```python
from build123d import *

# Parameters (mm, degrees)
SKETCH1_W           = 95.25
SKETCH1_H           = 101.6
BOSS_EXTRUDE1_DEPTH = 3.175
SKETCH5_R           = 0.99949
CUT_EXTRUDE3_DEPTH  = 3.175
CIRPATTERN3_COUNT   = 2
FILLET1_R           = 2.54
CHAMFER1_SIZE       = 1.27


with BuildPart() as part:
    # Sketch1 → Boss-Extrude1 (new body)
    with BuildSketch(Plane(origin=(0, 0, 0), x_dir=(1, 0, 0), z_dir=(0, 1, 0))):
        Rectangle(SKETCH1_W, SKETCH1_H)
    extrude(amount=BOSS_EXTRUDE1_DEPTH)

    # Sketch5 → Cut-Extrude3 (cut)
    with BuildSketch(Plane(origin=(0, 3.175, 0), x_dir=(1, 0, 0), z_dir=(0, 1, 0))):
        with Locations((-38.1, -44.45)):
            Circle(SKETCH5_R)
        with Locations((38.1, -44.45)):
            Circle(SKETCH5_R)
    cut_extrude3 = extrude(amount=-CUT_EXTRUDE3_DEPTH, mode=Mode.SUBTRACT)

    # CirPattern3: Cut-Extrude3 ×2 about axis
    cirpattern3_axis = Axis((0, 0, 0), (0, 1, 0))
    for i in range(1, CIRPATTERN3_COUNT):
        add(cut_extrude3.rotate(cirpattern3_axis, i * 360 / CIRPATTERN3_COUNT), mode=Mode.SUBTRACT)

    # Fillet1
    fillet1_edges = [part.edges().sort_by_distance(p)[0] for p in [
        (47.625, 3.175, 0),
        (0, 3.175, -50.8),
        (-47.625, 3.175, 0),
        (-47.625, 1.5875, -50.8),
        (47.625, 1.5875, -50.8),
        (47.625, 1.5875, 50.8),
        (-47.625, 1.5875, 50.8),
        (0, 3.175, 50.8),
    ]]
    fillet(fillet1_edges, radius=FILLET1_R)

    # Chamfer1
    chamfer1_edges = [part.edges().sort_by_distance(p)[0] for p in [
        (-39.09949, 0, 44.45),
        (37.10051, 0, 44.45),
        (39.09949, 0, -44.45),
        (-37.10051, 0, -44.45),
    ]]
    chamfer(chamfer1_edges, length=CHAMFER1_SIZE)


solid = part.part
```
Geometry: final body of the model. Coordinates: model frame, mm. Round coordinates to 2 decimals unless told otherwise and drop trailing zeros. Use one line per item in the form item = value.
(1) Ray query, probe 1 along X at (y, z) = (1.95, 44.45); probe 2 along Z at (x, y) = (38.1, 2.6); probe 3 along Z at (x, y) = (-38.1, 2.25). Return the intervals inside material, ascending. Write a range as [from, to].
Results list:
probe_1 = [-47.26, -39.1], [-37.1, 37.1], [39.1, 47.26]
probe_2 = [-49.87, -45.45], [-43.45, 43.45], [45.45, 49.87]
probe_3 = [-50.22, -45.45], [-43.45, 43.45], [45.45, 50.22]
(2) Section A-A on y = 2.6. Count the separate pieces of the cut face and the enclosed holes in it, and give its area (3 significant figures).
Results list:
separate_pieces = 1
enclosed_holes = 4
area = 9,300 mm^2
(3) First-contact query: pin 1 Ø1.5 at (y, z) = (2, -39.5) entering from -X. Flat tip, straight axial feed; report the tip coordinate or a pass-through.
Results list:
pin_1 = -47.55
